Build history of the part. All positions in model axes, mm. Face numbers are marked on the shaded views. A direction names the side the tool comes from. Round coordinates to 2 decimals unless told otherwise and drop trailing zeros. Write each loop counter-clockwise with the first axis right and the second up, starting at its lowest first coordinate (ties: lowest second). Pieces come first, ordered by that corner, then holes. Notation, with made-up numbers: (87.25, 72) - (108.25, 72) arc R21 cw to (108.25, 110) - close; hole circle Ø4 at (-38, -15.75). An arc over 180 degrees is marked (long way). Answer as a JSON object with one key per item and string values. Group by question number.
Item 1: Which spindle directions (+Z, -Z, +X, -X, +Y, -Y) get a long thin tool onto all of the face, cutting with end or side? Do the marked faces 4, 5, 6, 7 and 8. Say none if no direction does.
Item 2: Slice it at A-A, the plane y = -22.5. List the corners of the cut face in (x, z), then the cut area to 3 significant figures.
Item 3: Slice it at B-B, the plane y = -81. List the corners of the cut face in (x, z), then the cut area to 3 significant figures.
Item 4: Probe line 1 (Y direction, x = 60, z = 104.5); line 2 (X direction, y = -5.5, z = 6.5); line 3 (Y direction, x = 47, z = 102). List the from-to ranges inside material, lowest first. Write a range as from..to.
Item 5: Flat gauge pins, fed straight in: pin 1 (1.5 mm diameter, centred on y = -69.5, z = 110.5, fed in from +X); pin 2 (8 mm diameter, centred on x = -6, y = -17, fed in from +Z); pin 3 (3.5 mm diameter, centred on x = 30.5, z = 91.5, fed in from +Y). Where does each tip first touch, or does it go through?
Item 6: Slice it at C-C, the plane y = -49.5. List the corners of the cut face in (x, z).
Item 7: Two-plate mould, pull along X, no slides. Class the marked faces 1, 2 and 3: +X half, -X half, draft (parallel to the pull), parting line (faces both ways), or undercut.
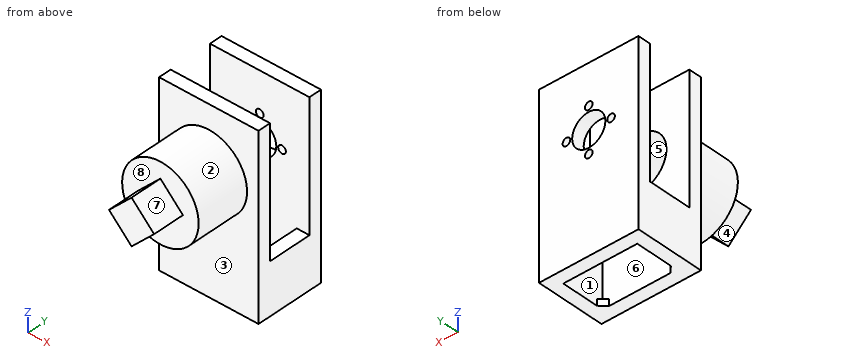
from build123d import *

# Parameters (mm, degrees)
SKETCH_1_W               = 78
SKETCH_1_H               = 54.155555556
SKETCH_1_W_2             = 58
SKETCH_1_H_2             = 34.155555556
EXTRUDE_1_DEPTH          = 40
SKETCH_2_W               = 78
SKETCH_2_H               = 10
EXTRUDE_1_2_DEPTH        = 100
EXTRUDE_2_DEPTH          = 5
SKETCH_4_R               = 21
CUT_EXTRUDE_1_DEPTH      = 162.782919637
EXTRUDE_3_DEPTH          = 100
CUT_EXTRUDE_2_REACH      = 166.793
SKETCH_6_R               = 13
SKETCH_8_R               = 3
CUT_EXTRUDE_3_DEPTH      = 35
PATTERN_CIRCULAR_1_COUNT = 4
SKETCH_9_R               = 30
SKETCH_9_R_2             = 21
EXTRUDE_4_DEPTH          = 22
SKETCH_10_R              = 30
SKETCH_10_R_2            = 3.5
EXTRUDE_5_DEPTH          = 20
EXTRUDE_6_DEPTH          = 25


with BuildPart() as part:
    # 草图1 → Extrude 1 (new body)
    with BuildSketch(Plane.XY):
        with Locations((29, -17.077777778)):
            Rectangle(SKETCH_1_W, SKETCH_1_H)
        with Locations((29, -17.077777778)):
            Rectangle(SKETCH_1_W_2, SKETCH_1_H_2, mode=Mode.SUBTRACT)
    extrude(amount=EXTRUDE_1_DEPTH)

    # 草图2 → Extrude 1 2 (add)
    with BuildSketch(Plane.XY.offset(40)):
        with Locations((29, -39.155555556)):
            Rectangle(SKETCH_2_W, SKETCH_2_H)
    extrude(amount=EXTRUDE_1_2_DEPTH)

    # 草图3 → 凸台-拉伸2 (add)
    with BuildSketch(Plane(origin=(0, 0, 0), x_dir=(-1, 0, 0), z_dir=(0, 0, -1))):
        Polygon((-58, -29.155555556), (-58, -34.155555556), (-53, -34.155555556), align=None)
        Polygon((0, -29.155555556), (0, -34.155555556), (-5, -34.155555556), align=None)
    extrude(amount=-EXTRUDE_2_DEPTH)

    # 草图4 → 切除-拉伸1 (cut, through all)
    with BuildSketch(Plane(origin=(0, -34.155555556, 0), x_dir=(1, 0, 0), z_dir=(0, 1, 0))):
        with Locations(Location((29, -91.398483043, 0), (0, 0, 270))):
            Circle(SKETCH_4_R)
    extrude(amount=-CUT_EXTRUDE_1_DEPTH, mode=Mode.SUBTRACT)

    # 草图5 → 凸台-拉伸3 (add)
    with BuildSketch(Plane.XY.offset(40)):
        Polygon((-10, 10), (-10, 0), (0, 0), (58, 0), (68, 0), (68, 10), align=None)
    extrude(amount=EXTRUDE_3_DEPTH)

    # 草图6 → 切除-拉伸2 (cut, up to next)
    with BuildSketch(Plane(origin=(0, 10, 0), x_dir=(1, 0, 0), z_dir=(0, 1, 0)), mode=Mode.PRIVATE) as cut_extrude_2_sk1:
        with Locations(Location((29, -91.398483043, 0), (0, 0, 270))):
            Circle(SKETCH_6_R)
    cut_extrude_2_tool1 = extrude(cut_extrude_2_sk1.sketch, amount=-CUT_EXTRUDE_2_REACH, mode=Mode.PRIVATE) & part.part
    add(cut_extrude_2_tool1.solids().sort_by_distance((29, 10, 91.398483))[0], mode=Mode.SUBTRACT)

    # 草图8 → 切除-拉伸3 (cut)
    with BuildSketch(Plane(origin=(0, 10, 0), x_dir=(1, 0, 0), z_dir=(0, 1, 0))):
        with Locations(Location((29, -73.898483043, 0), (0, 0, 270))):
            Circle(SKETCH_8_R)
    cut_extrude_3 = extrude(amount=-CUT_EXTRUDE_3_DEPTH, mode=Mode.SUBTRACT)

    # 阵列(圆周)1: 切除-拉伸3 ×4 about axis
    pattern_circular_1_axis = Axis((29, 0, 91.398483043), (0, 1, 0))
    for i in range(1, PATTERN_CIRCULAR_1_COUNT):
        add(cut_extrude_3.rotate(pattern_circular_1_axis, i * 360 / PATTERN_CIRCULAR_1_COUNT), mode=Mode.SUBTRACT)

    # 草图9 → 凸台-拉伸4 (add)
    with BuildSketch(Plane.XZ.offset(44.155555556)):
        with Locations(Location((29, 91.398483043, 0), (0, 0, 90))):
            Circle(SKETCH_9_R)
        with Locations(Location((29, 91.398483043, 0), (0, 0, 90))):
            Circle(SKETCH_9_R_2, mode=Mode.SUBTRACT)
    extrude(amount=EXTRUDE_4_DEPTH)

    # 草图10 → 凸台-拉伸5 (add)
    with BuildSketch(Plane.XZ.offset(66.155555556)):
        with Locations(Location((29, 91.398483043, 0), (0, 0, 90))):
            Circle(SKETCH_10_R)
        with Locations(Location((29, 91.398483043, 0), (0, 0, 270))):
            Circle(SKETCH_10_R_2, mode=Mode.SUBTRACT)
    extrude(amount=EXTRUDE_5_DEPTH)

    # 草图12 → 凸台-拉伸6 (add)
    with BuildSketch(Plane.XZ.offset(86.155555556)):
        Polygon((11.32233047, 91.398483043), (29, 109.076152573), (46.67766953, 91.398483043), (29, 73.720813513), align=None)
    extrude(amount=EXTRUDE_6_DEPTH)


solid = part.part
Geometry says:
{
 "1": {"face 4": "-Z, -X, -Y", "face 5": "none", "face 6": "+Z", "face 7": "+Z, +X, -Y", "face 8": "-Y"},
 "2": {"outline": "(-10, 0) - (0, 0) - (0, 40) - (-10, 40) - close; (58, 0) - (68, 0) - (68, 40) - (58, 40) - close", "area": "800 mm^2"},
 "3": {"outline": "circle Ø60 at (29, 91.4); hole circle Ø7 at (29, 91.4)", "area": "2,790 mm^2"},
 "4": {"line 1": "y = -44.16..-34.16, 0..10", "line 2": "x = -10..0, 58..68", "line 3": "y = -86.16..-66.16, 0..10"},
 "5": {"pin 1": "stops at x = 52.73", "pin 2": "stops at z = 40", "pin 3": "stops at y = -86.16"},
 "6": {"outline": "circle Ø60 at (29, 91.4); hole circle Ø42 at (29, 91.4)"},
 "7": {"face 1": "undercut", "face 2": "parting line", "face 3": "draft"}
}
